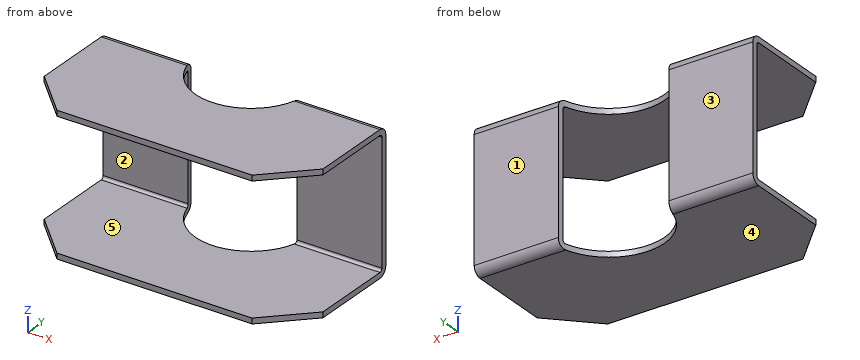
from build123d import *

# Parameters (mm, degrees)
F1_DEPTH      = 100
F1_DEPTH_BACK = 100
F2_R          = 40
F3_DEPTH      = 100
F3_DEPTH_BACK = 100
F4_SIZE       = 30


with BuildPart() as f1:
    # F0 (on Right) → F1 (new body, two sides)
    with BuildSketch(Plane.YZ) as f1_sk:
        with BuildLine():
            Line((-5, 0), (-5, 44))
            ThreePointArc((-5, 44), (-6.757359, 48.242641), (-11, 50))
            Line((-11, 50), (-100, 50))
            Line((-100, 50), (-100, 46))
            Line((-100, 46), (-11, 46))
            ThreePointArc((-11, 46), (-9.585786, 45.414214), (-9, 44))
            Line((-9, 44), (-9, 0))
            Line((-9, 0), (-9, -44))
            ThreePointArc((-9, -44), (-9.585786, -45.414214), (-11, -46))
            Line((-11, -46), (-100, -46))
            Line((-100, -46), (-100, -50))
            Line((-100, -50), (-11, -50))
            ThreePointArc((-11, -50), (-6.757359, -48.242641), (-5, -44))
            Line((-5, -44), (-5, 0))
        make_face()
    extrude(amount=F1_DEPTH)
    extrude(f1_sk.sketch, amount=-F1_DEPTH_BACK)

    # F2 (on Top) → F3 (cut, two sides)
    with BuildSketch(Plane.XY) as f3_sk:
        Circle(F2_R)
    extrude(amount=F3_DEPTH, mode=Mode.SUBTRACT)
    extrude(f3_sk.sketch, amount=-F3_DEPTH_BACK, mode=Mode.SUBTRACT)

    # F4
    f4_edges = [f1.edges().sort_by_distance(p)[0] for p in [
        (100, -100, -48),
        (100, -100, 48),
        (-100, -100, -48),
        (-100, -100, 48),
    ]]
    chamfer(f4_edges, length=F4_SIZE)


solid = f1.part
Source: CAD feature listing. Evaluate the final solid. Frame: model axes, mm. Face numbers are marked on the shaded views. A direction names the side the tool comes from. Give positions to 0.01 mm unless a question says otherwise; leave off trailing zeros. Write each loop counter-clockwise with the first axis right and the second up, starting at its lowest first coordinate (ties: lowest second). Pieces come first, ordered by that corner, then holes. Notation, with made-up numbers: M 77.25,69.5 L 124.25,69.5 A23 ccw 124.25,97.5 Z; hole C 63,80 d8. An arc over 180 degrees is marked long. Answer as a JSON object with one key per item and string values.
Q1. Cut plane B-B, the plane z = -12.5. Return the cut outline in (x, y), then the cut area to 3 significant figures.
Geometry check:
{"outline": "M -100,-9 L -38.97,-9 A40 cw -39.69,-5 L -100,-5 Z; M 38.97,-9 L 100,-9 L 100,-5 L 39.69,-5 A40 cw Z", "area": "485 mm^2"}
Q2. Access query for the marked faces 1 and 2. Directions: +Z, -Z, +X, -X, +Y, -Y. A direction counts if a zero-diameter tool reaches every point of the face in a straight line with its end or side. Return the directions, or none.
Geometry check:
{"face 1": "+Z, -Z, +X, -X, +Y", "face 2": "+X, -X, -Y"}
Q3. Cut plane D-D, the plane y = -28. Return the cut outline in (x, z).
Geometry check:
{"outline": "M -100,-50 L -28.57,-50 L -28.57,-46 L -100,-46 Z; M -100,46 L -28.57,46 L -28.57,50 L -100,50 Z; M 28.57,-50 L 100,-50 L 100,-46 L 28.57,-46 Z; M 28.57,46 L 100,46 L 100,50 L 28.57,50 Z"}
Q4. Ray query, line 1 along Z through (x, y) = (-49, -30.5); line 2 along Y through (x, z) = (47, -23); line 3 along Z through (x, y) = (46, -8.5). Return the intervals inside material, ascending.
Geometry check:
{"line 1": "z = -50 to -46, 46 to 50", "line 2": "y = -9 to -5", "line 3": "z = -49.45 to 49.45"}
Q5. Mould query, pull axis Z, two halves, no side actions, for the marked faces 3, 4 and 5. Classes: +Z half, -Z half, draft (parallel to the pull), parting line (faces both ways), or undercut.
Geometry check:
{"face 3": "draft", "face 4": "-Z half", "face 5": "undercut"}
Q6. Cut plane A-A, the plane y = -79.5. Return the cut outline in (x, z).
Geometry check:
{"outline": "M -90.5,-50 L 90.5,-50 L 90.5,-46 L -90.5,-46 Z; M -90.5,46 L 90.5,46 L 90.5,50 L -90.5,50 Z"}
Q7. Cut plane C-C, the plane x = -74.5. Return the cut outline in (y, z), then the cut area to 3 significant figures.
Geometry check:
{"outline": "M -95.5,-50 L -11,-50 A6 ccw -5,-44 L -5,44 A6 ccw -11,50 L -95.5,50 L -95.5,46 L -11,46 A2 cw -9,44 L -9,-44 A2 cw -11,-46 L -95.5,-46 Z", "area": "1,080 mm^2"}
